Part model, mm, in its own coordinate system. Face numbers are marked on the shaded views. A direction names the side the tool comes from. Coordinates: 2 decimals unless noted, no trailing zeros. Write each loop counter-clockwise with the first axis right and the second up, starting at its lowest first coordinate (ties: lowest second). Pieces come first, ordered by that corner, then holes. Notation, with made-up numbers: (21.25, -10.5) -> (41.25, -10.5) arc R19 cw to (41.25, -0.5) -> close; hole circle Ø4 at (4, -26.5). An arc over 180 degrees is marked (long way). Write item = value, one per line. Start each with the question number.
Q1. Pin check, flat tips, straight feed: P1, Ø3.5, axis at x = 4.5, y = 18, coming from the +Z side; P2, Ø0.9, axis at x = 3.5, z = -18, coming from the -Y side; P3, Ø3.5, axis at x = 3, y = -18, coming from the +Z side. Stop position of each tip, or through.
Q2. Band-saw the part on B-B, the plane y = -10.5. List the corners of the cut face in (x, z).
Q3. Pull direction Y, two halves, no side cores. Call the marked faces 1, 2, 3 and 4: released by +Y, released by -Y, zero draft, split by the parting line, or undercut.
Q4. Band-saw the part on A-A, the plane z = 1. List the corners of the cut face in (x, y) (3 decimals).
Q5. Probe line 1 (Y direction, x = 5.5, z = -16.5); line 2 (Y direction, x = 2, z = -12). List the from-to ranges inside material, lowest first.
Q6. Tool access for the marked faces 5, 6, 7 and 8: list every direction of +Z, -Z, +X, -X, +Y, -Y with a clear straight run to the whole face (end or side of a thin tool).
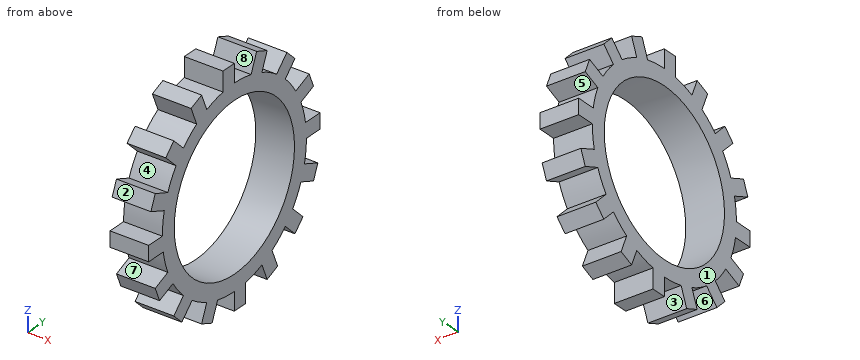
Autodesk Inventor part; units mm, degrees
ref_plane "YZ Plane" through (0, 0, 0) normal (1, 0, 0) x (0, 1, 0)
ref_plane "XZ Plane" through (0, 0, 0) normal (0, 1, 0) x (-1, 0, 0)
ref_plane "XY Plane" through (0, 0, 0) normal (0, 0, 1) x (1, 0, 0)
sketch "Sketch1" plane through (0, 0, 0) normal (1, 0, 0) x (0, 1, 0)
  circle A0 centre (0, 0) radius 13.25
  circle A1 centre (0, 0) radius 15.875
  line L0 (15.875, 0) -> (18.875, 0)
  line L1 (18.875, 0) -> (18.875, 2.5)
  line L2 (18.875, 2.5) -> (15.6769, 2.5)
  line L3 (17.4382, 7.2231) -> (16.4815, 9.5328)
  line L4 (16.4815, 9.5328) -> (13.5269, 8.309)
  line L5 (14.6666, 6.0751) -> (17.4382, 7.2231)
  line L6 (13.3466, 13.3466) -> (11.5789, 15.1144)
  line L7 (11.5789, 15.1144) -> (9.3175, 12.853)
  line L8 (11.2253, 11.2253) -> (13.3466, 13.3466)
  line L9 (7.2231, 17.4382) -> (4.9135, 18.3949)
  line L10 (4.9135, 18.3949) -> (3.6896, 15.4403)
  line L11 (6.0751, 14.6666) -> (7.2231, 17.4382)
  line L12 (0, 18.875) -> (-2.5, 18.875)
  line L13 (-2.5, 18.875) -> (-2.5, 15.6769)
  line L14 (0, 15.875) -> (0, 18.875)
  line L15 (-7.2231, 17.4382) -> (-9.5328, 16.4815)
  line L16 (-9.5328, 16.4815) -> (-8.309, 13.5269)
  line L17 (-6.0751, 14.6666) -> (-7.2231, 17.4382)
  line L18 (-13.3466, 13.3466) -> (-15.1144, 11.5789)
  line L19 (-15.1144, 11.5789) -> (-12.853, 9.3175)
  line L20 (-11.2253, 11.2253) -> (-13.3466, 13.3466)
  line L21 (-17.4382, 7.2231) -> (-18.3949, 4.9135)
  line L22 (-18.3949, 4.9135) -> (-15.4403, 3.6896)
  line L23 (-14.6666, 6.0751) -> (-17.4382, 7.2231)
  line L24 (-18.875, 0) -> (-18.875, -2.5)
  line L25 (-18.875, -2.5) -> (-15.6769, -2.5)
  line L26 (-15.875, 0) -> (-18.875, 0)
  line L27 (-17.4382, -7.2231) -> (-16.4815, -9.5328)
  line L28 (-16.4815, -9.5328) -> (-13.5269, -8.309)
  line L29 (-14.6666, -6.0751) -> (-17.4382, -7.2231)
  line L30 (-13.3466, -13.3466) -> (-11.5789, -15.1144)
  line L31 (-11.5789, -15.1144) -> (-9.3175, -12.853)
  line L32 (-11.2253, -11.2253) -> (-13.3466, -13.3466)
  line L33 (-7.2231, -17.4382) -> (-4.9135, -18.3949)
  line L34 (-4.9135, -18.3949) -> (-3.6896, -15.4403)
  line L35 (-6.0751, -14.6666) -> (-7.2231, -17.4382)
  line L36 (0, -18.875) -> (2.5, -18.875)
  line L37 (2.5, -18.875) -> (2.5, -15.6769)
  line L38 (0, -15.875) -> (0, -18.875)
  line L39 (7.2231, -17.4382) -> (9.5328, -16.4815)
  line L40 (9.5328, -16.4815) -> (8.309, -13.5269)
  line L41 (6.0751, -14.6666) -> (7.2231, -17.4382)
  line L42 (13.3466, -13.3466) -> (15.1144, -11.5789)
  line L43 (15.1144, -11.5789) -> (12.853, -9.3175)
  line L44 (11.2253, -11.2253) -> (13.3466, -13.3466)
  line L45 (17.4382, -7.2231) -> (18.3949, -4.9135)
  line L46 (18.3949, -4.9135) -> (15.4403, -3.6896)
  line L47 (14.6666, -6.0751) -> (17.4382, -7.2231)
  dimension "d1" = 31.75
  dimension "d0" = 26.5
  dimension "d3" = 3
  dimension "d4" = 2.5
  dimension "d7" = 360
extrude "Extrusion1" add sketch "Sketch1" along normal blind 6.35
properties part number "wedge holder" material "ABS Plastic"
Ans:
q1.P1 = 9.53
q1.P2 = -6.95
q1.P3 = 7.22
q2.outline = (0, -14.04) -> (6.35, -14.04) -> (6.35, -8.08) -> (0, -8.08) -> close; (0, 8.08) -> (6.35, 8.08) -> (6.35, 11.91) -> (0, 11.91) -> close
q3.face_1 = zero draft
q3.face_2 = released by -Y
q3.face_3 = undercut
q3.face_4 = undercut
q4.outline = (0, -15.843) -> (6.35, -15.843) -> (6.35, -13.212) -> (0, -13.212) -> close; (0, 13.212) -> (6.35, 13.212) -> (6.35, 18.875) -> (0, 18.875) -> close
q5.line_1 = -6.83 to -4.13, 0 to 2.5, 6.83 to 9.49
q5.line_2 = -12 to -5.62, 5.62 to 10.39, 12 to 14.69
q6.face_5 = +X, -X, +Y
q6.face_6 = -Z, +X, -X
q6.face_7 = +X, -X, -Y
q6.face_8 = +Z, +X, -X
